Design review of the part built by this model. Coordinates are the model's own, in mm. Face numbers are marked on the shaded views. Give positions to 0.01 mm unless a question says otherwise; leave off trailing zeros.
from build123d import *

# Parameters (mm, degrees)
F1_DEPTH = 5


with BuildPart() as f1:
    # F0 (on Top) → F1 (new body)
    with BuildSketch(Plane.XY):
        with BuildLine():
            add(Edge.make_bspline(
                [(90.6907990575, 97.9469045997), (92.5506797048, 97.7076608643), (97.3714835458, 97.0875419767), (111.3982823465, 88.6117833473), (121.080150162, 80.1037886779), (126.2320578098, 75.5765214562)],
                knots=[0, 0, 0, 0, 0.2271401523, 0.5887464448, 1, 1, 1, 1], degree=3))
            Line((90.6907990575, 97.9469045997), (85.0284695625, 83.2098796964))
            Line((85.0284695625, 83.2098796964), (40.8717952669, 72.0387473702))
            add(Edge.make_bspline(
                [(40.8717952669, 72.0387473702), (39.4639939865, 69.9245000162), (37.1445701485, 66.4411705287), (33.9493519923, 64.4696102192), (29.6565838044, 68.4823153989), (29.2317022817, 78.7511303066), (28.945825994, 85.6603756547)],
                knots=[0, 0, 0, 0, 0.2489757455, 0.4102001378, 0.6031604435, 1, 1, 1, 1], degree=3))
            Line((28.945825994, 85.6603756547), (18.8582092524, 76.4733627439))
            add(Edge.make_bspline(
                [(-18.1637965143, 76.4733627439), (-14.1437358291, 77.1075253303), (-6.0536026016, 78.3837398489), (6.5737675387, 78.534699391), (14.7693251616, 77.1594799333), (18.8582092524, 76.4733627439)],
                knots=[0, 0, 0, 0, 0.331071517, 0.6662617533, 1, 1, 1, 1], degree=3))
            Line((-18.1637965143, 76.4733627439), (-28.2951612025, 85.8325883746))
            add(Edge.make_bspline(
                [(-40.3230860829, 72.0387473702), (-39.088224818, 70.1720803209), (-37.0503190798, 67.0914982353), (-35.1522700417, 65.3354549205), (-31.9776770355, 64.7647193737), (-30.3977678177, 67.0311278125), (-28.4521818074, 74.4454913779), (-28.3514925601, 81.747451692), (-28.2951612025, 85.8325883746)],
                knots=[0, 0, 0, 0, 0.183795483, 0.303319798, 0.4263136272, 0.5389125099, 0.7420411316, 1, 1, 1, 1], degree=3))
            Line((-40.3230860829, 72.0387473702), (-84.1391906142, 83.2098796964))
            Line((-84.1391906142, 83.2098796964), (-90.1290997863, 97.9469045997))
            add(Edge.make_bspline(
                [(-90.1290997863, 97.9469045997), (-91.2780209136, 97.8755945292), (-94.8799122656, 97.6520359926), (-112.2832793798, 87.9203392551), (-121.5116369775, 79.7034292861), (-126.1465400457, 75.5765214562)],
                knots=[0, 0, 0, 0, 0.1890607113, 0.5927092164, 1, 1, 1, 1], degree=3))
            add(Edge.make_bspline(
                [(-126.1465400457, 75.5765214562), (-132.559519944, 69.6540069441), (-147.2325322521, 56.1031881811), (-173.7268363632, 15.3201798146), (-185.3013561139, -10.9793593897), (-194.7659689395, -44.6073790263), (-195.2399434774, -52.7711224043), (-195.410117507, -55.7022020221)],
                knots=[0, 0, 0, 0, 0.1990617008, 0.4554567194, 0.6642768347, 0.8794632215, 1, 1, 1, 1], degree=3))
            add(Edge.make_bspline(
                [(-195.410117507, -55.7022020221), (-189.2443233147, -51.3534252403), (-176.6787449134, -42.490836919), (-153.3171130308, -33.7752578796), (-140.3890181065, -30.5398782143), (-134.3097835779, -29.0184915066)],
                knots=[0, 0, 0, 0, 0.3379220853, 0.6886682111, 1, 1, 1, 1], degree=3))
            Line((-134.3097835779, -29.0184915066), (-125.7226914167, -37.7225726843))
            Line((-125.7226914167, -37.7225726843), (-115.6381219625, -27.0764511079))
            add(Edge.make_bspline(
                [(-115.6381219625, -27.0764511079), (-112.3214448117, -25.6089260502), (-105.9657828163, -22.7967460241), (-97.1811480846, -21.5375744889), (-87.7828374292, -23.7605556506), (-84.2924143647, -26.0591359078), (-82.7476084232, -27.0764511079)],
                knots=[0, 0, 0, 0, 0.2773913223, 0.5315577625, 0.7926748883, 1, 1, 1, 1], degree=3))
            Line((-82.7476084232, -27.0764511079), (0, -73.3860805631))
            Line((0, -73.3860805631), (0.147642626, -73.3210891485))
            Line((0.147642626, -73.3210891485), (64.6225735545, -37.7225726843))
            add(Edge.make_bspline(
                [(64.6225735545, -37.7225726843), (73.0666381112, -32.529493092), (87.0501240706, -23.9296825297), (99.0743607688, -21.6967578796), (108.2136687045, -23.3658879949), (113.2473852724, -25.8509101796), (115.729868412, -27.0764511079)],
                knots=[0, 0, 0, 0, 0.3591296563, 0.5947236041, 0.800129426, 1, 1, 1, 1], degree=3))
            Line((115.729868412, -27.0764511079), (125.9138733149, -37.7225726843))
            Line((125.9138733149, -37.7225726843), (135.1518183947, -29.0184915066))
            add(Edge.make_bspline(
                [(196.0572302341, -55.7022020221), (192.7366020121, -53.1840689017), (185.2187189114, -47.4830300727), (166.9431190304, -38.1587419464), (145.4004429365, -31.4769398334), (138.082034766, -29.7213941747), (135.1518183947, -29.0184915066)],
                knots=[0, 0, 0, 0, 0.2245071862, 0.508282972, 0.8031214914, 1, 1, 1, 1], degree=3))
            add(Edge.make_bspline(
                [(126.2320578098, 75.5765214562), (134.7565386666, 67.382737054), (151.0099741889, 51.7598330082), (166.021851899, 28.1874163152), (182.5105457126, -0.6670200083), (190.1905976163, -26.8526885409), (194.0803362932, -45.9807089416), (196.0572302341, -55.7022020221)],
                knots=[0, 0, 0, 0, 0.2126150187, 0.4053882641, 0.6130102113, 0.8033189805, 1, 1, 1, 1], degree=3))
        make_face()
    extrude(amount=F1_DEPTH)


solid = f1.part
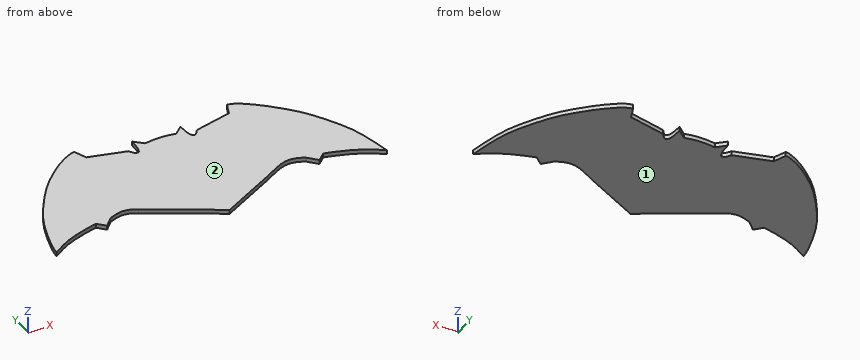
Q1. Draft analysis for pull direction Z (two halves, no side actions). For the marked faces 1 and 2, state which applies: pulls with the +Z half, pulls with the -Z half, needs draft (parallel to the pull), parting line crosses it, or undercut.
Results:
face 1: pulls with the -Z half
face 2: pulls with the +Z half
Q2. Wall thickness on line 1 (X direction, y = -45.5, z = 3.75); line 2 (Y direction, x = -15, z = 3.25); line 3 (Y direction, x = 94, z = 2.45): over which ranges is each line inside the solid? List them lowest first.
Results:
line 1: x = -194.25 to -179.98, -49.83 to 50.54, 180.86 to 193.97
line 2: y = -64.99 to 76.97
line 3: y = -22.84 to 97.41
Q3. Insertion check: pin 1 (4 mm diameter, centred on x = 129.5, y = 73, fed in from -Z); pin 2 (1.5 mm diameter, centred on x = -139, z = 1.5, fed in from -Y). Each pin has a flat end and moves straight along its axis. Give the tip position at first contact, or say it passes through.
Results:
pin 1: stops at z = 0
pin 2: stops at y = -30.39
Q4. Take a section at A-A (y = -43). Give the number of separate pieces and of enclosed holes in the cut face, plus the area to 3 significant figures.
Results:
separate pieces: 3
enclosed holes: 0
area: 725 mm2
